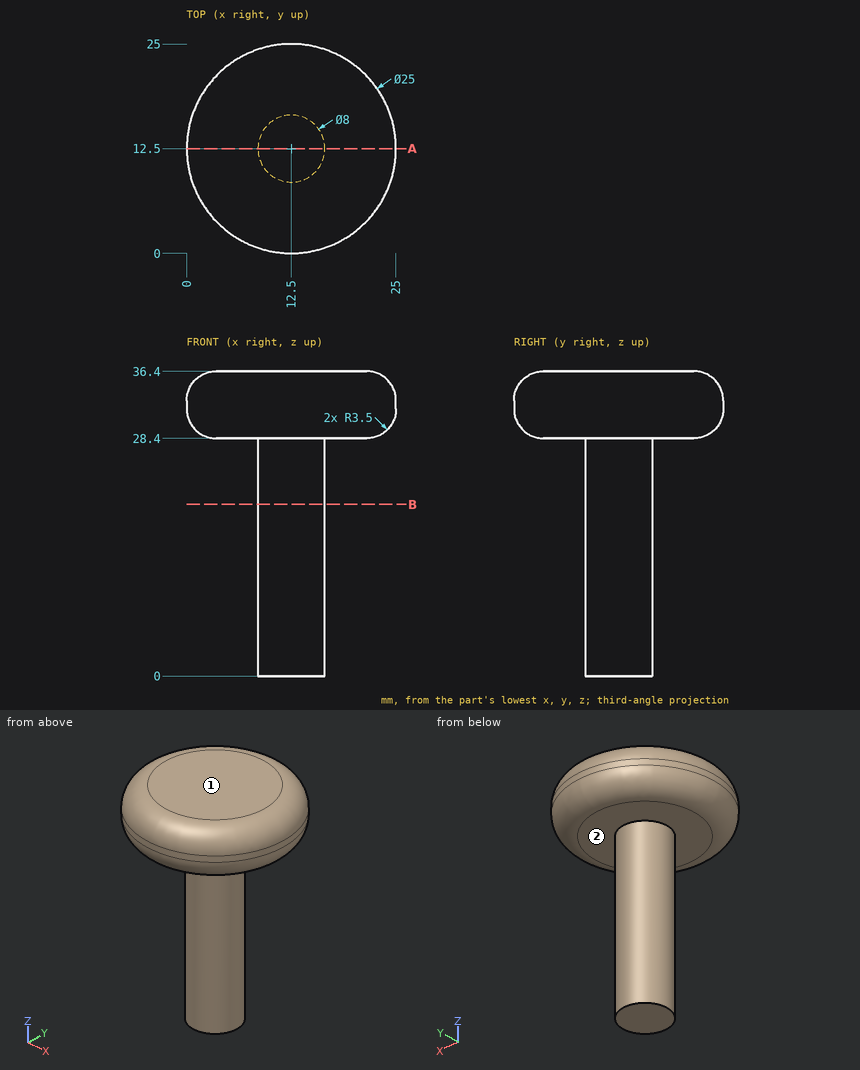
Answer from the drawing. Dimensions are ordinates in mm from the lowest x, y and z of the part. A direction names the side the tool comes from. Give positions to 0.01 mm unless a question says otherwise; leave off trailing zeros. Loops run counter-clockwise (first coordinate to the right, second up) from the corner with the lowest first, then second, coordinate; pieces in that order, holes last. Notation, with made-up numbers: (16.25, 41) - (41.25, 41) arc R27 ccw to (41.25, 60) - close; hole circle Ø6 at (64.5, 3). An arc over 180 degrees is marked (long way). Answer as a JSON object with one key per item and string values.
1. A cutting plane is placed at A-A (y = 12.5). Write down the section's boundary in (x, z), then the cut area to 3 significant figures.
Determined:
{"outline": "(0, 31.9) arc R3.5 ccw to (3.5, 28.4) - (8.5, 28.4) - (8.5, 0) - (16.5, 0) - (16.5, 28.4) - (21.5, 28.4) arc R3.5 ccw to (25, 31.9) - (25, 32.9) arc R3.5 ccw to (21.5, 36.4) - (3.5, 36.4) arc R3.5 ccw to (0, 32.9) - close", "area": "417 mm²"}
2. Flat-ended cylindrical pins translate along their axes: pin 1 Ø1.5 at (x, y) = (21.5, 4.5) entering from +Z; pin 2 Ø10 at (x, y) = (10.5, 3.5) entering from +Z; pin 3 Ø8 at (x, z) = (9, 6) entering from -Y; pin 4 Ø6 at (x, z) = (3.5, 24.5) entering from -Y. Find the tip coordinate at first contact, or state that the pin passes through.
Determined:
{"pin 1": "z = 35.55", "pin 2": "z = 36.4", "pin 3": "y = 8.5", "pin 4": "through"}
3. A cutting plane is placed at B-B (z = 20.5). Write down the section's boundary in (x, y), then the cut area to 3 significant figures.
Determined:
{"outline": "circle Ø8 at (12.5, 12.5)", "area": "50.3 mm²"}
4. Find the intervals of material crossed by L1, parallel to Z at x = 13.75, y = 17.25; L2, parallel to Y at x = 12.25, z = 20; L3, parallel to Y at x = 19.5, z = 30.5, in increasing order. Write a range as [from, to].
Determined:
{"L1": "[28.4, 36.4]", "L2": "[8.51, 16.49]", "L3": "[2.5, 22.5]"}
5. For the marked faces 1 and 2, determine the directions among +Z, -Z, +X, -X, +Y, -Y from which every point of the face is accessible in a straight line to the end or side of a thin tool.
Determined:
{"face 1": "+Z, +X, -X, +Y, -Y", "face 2": "-Z"}
